Could you check a few things on this model? Use its own coordinates, in mm. A direction names the side the tool comes from. Coordinates: 2 decimals unless noted, no trailing zeros. Loops run counter-clockwise (first coordinate to the right, second up) from the corner with the lowest first, then second, coordinate; pieces in that order, holes last. Notation, with made-up numbers: (58.25, 33.25) -> (113.25, 33.25) arc R25 ccw to (113.25, 62.25) -> close; hole circle Ø9 at (79.25, -19.5). An arc over 180 degrees is marked (long way). One line per question, with ' | ' between items.
```python
from build123d import *

# Parameters (mm, degrees)
F0_W     = 32
F0_H     = 16
F1_DEPTH = 10
F2_R     = 2.5
F3_DEPTH = 2
F4_T     = -2
F5_R     = 3.75
F5_R_2   = 3.25
F6_DEPTH = 8
F8_DEPTH = 6.5


with BuildPart() as f1:
    # F0 (on Top) → F1 (new body)
    with BuildSketch(Plane.XY):
        Rectangle(F0_W, F0_H)
    extrude(amount=F1_DEPTH)

    # F2 (on face) → F3 (join)
    with BuildSketch(Plane.XY.offset(10)):
        with Locations((-11.5, 4)):
            Circle(F2_R)
        with Locations((-3.5, 4)):
            Circle(F2_R)
        with Locations((12.5, 4)):
            Circle(F2_R)
        with Locations((12.5, -4)):
            Circle(F2_R)
        with Locations((4.5, -4)):
            Circle(F2_R)
        with Locations((-3.5, -4)):
            Circle(F2_R)
        with Locations((-11.5, -4)):
            Circle(F2_R)
        with Locations((4.5, 4)):
            Circle(F2_R)
    extrude(amount=F3_DEPTH)

    # F4
    f4_openings = [f1.faces().sort_by_distance(p)[0] for p in [
        (0, 0, 0),
    ]]
    offset(amount=F4_T, openings=f4_openings, kind=Kind.INTERSECTION)

    # F5 (on face) → F6 (join, through all)
    with BuildSketch(Plane(origin=(0, 0, 8), x_dir=(1, 0, 0), z_dir=(0, 0, -1))):
        with Locations((-7.5, 0)):
            Circle(F5_R)
        with Locations((-7.5, 0)):
            Circle(F5_R_2, mode=Mode.SUBTRACT)
        with Locations((0.7, 0)):
            Circle(F5_R)
        with Locations((0.7, 0)):
            Circle(F5_R_2, mode=Mode.SUBTRACT)
        with Locations((8.9, 0)):
            Circle(F5_R)
        with Locations((8.9, 0)):
            Circle(F5_R_2, mode=Mode.SUBTRACT)
    extrude(amount=F6_DEPTH)

    # F7 (on face) → F8 (join)
    with BuildSketch(Plane(origin=(0, 0, 8), x_dir=(1, 0, 0), z_dir=(0, 0, -1))):
        with BuildLine():
            ThreePointArc((-1.3, 3.1721443851), (0.7, 3.75), (2.7, 3.1721443851))
            Line((2.7, 3.1721443851), (2.7, 6))
            Line((2.7, 6), (-1.3, 6))
            Line((-1.3, 6), (-1.3, 3.1721443851))
        make_face()
        with BuildLine():
            Line((2.7, -6), (2.7, -3.1721443851))
            ThreePointArc((2.7, -3.1721443851), (0.7, -3.75), (-1.3, -3.1721443851))
            Line((-1.3, -3.1721443851), (-1.3, -6))
            Line((-1.3, -6), (2.7, -6))
        make_face()
    extrude(amount=F8_DEPTH)


solid = f1.part
```
Q1. For faces 1 (the face through (-14, 4, 11)), 2 (the face through (-4, -4, 12)), 3 (the face through (-3.5, -4, 10)), which set-ups out of +Z, -Z, +X, -X, +Y, -Y let a thin tool reach every point of the face, with its end or its side?
Values follow:
face 1: +Z | face 2: +Z, +X, -X, +Y, -Y | face 3: -Z
Q2. We'd pull the mould along X, two halves only. Please class faces 4 (the face through (-2.064, -2.534, 4.056)), 5 (the face through (0, 7, 0)): released by +X, released by -X, zero draft, split by the parting line, or undercut.
Values follow:
face 4: undercut | face 5: zero draft
Q3. For pin 1 (3 mm diameter, centred on x = 1, y = -4.5, fed in from -Z); pin 2 (1.1 mm diameter, centred on x = 12.5, y = -4, fed in from -Z); pin 3 (0.5 mm diameter, centred on x = 4.5, y = 4, fed in from -Z), each with a flat end and sliding along its axis, tell me the tip position at first contact or that it passes through.
Values follow:
pin 1: stops at z = 0 | pin 2: stops at z = 8 | pin 3: stops at z = 10
Q4. Imagine slicing it at B-B on z = 10.5. Write out the boundary of the cut face in (x, y), plus the area to 3 significant figures.
Values follow:
outline: circle Ø5 at (-11.5, -4); circle Ø5 at (-11.5, 4); circle Ø5 at (-3.5, -4); circle Ø5 at (-3.5, 4); circle Ø5 at (4.5, -4); circle Ø5 at (4.5, 4); circle Ø5 at (12.5, -4); circle Ø5 at (12.5, 4) | area: 157 mm2
Q5. Please list where these lines run through material, in increasing order: L1, parallel to Y at x = 8.9, z = 2.5; L2, parallel to Y at x = 12.5, z = 9.05; L3, parallel to X at y = 4, z = 9.15. Write a range as [from, to].
Values follow:
L1: y = [-8, -6], [-3.75, -3.25], [3.25, 3.75], [6, 8] | L2: y = [-8, -4.5], [-3.5, 3.5], [4.5, 8] | L3: x = [-16, -12], [-11, -4], [-3, 4], [5, 12], [13, 16]
Q6. Imagine slicing it at A-A on z = 3.25. Write out the boundary of the cut face in (x, y).
Values follow:
outline: (-16, -8) -> (16, -8) -> (16, 8) -> (-16, 8) -> close; circle Ø7.5 at (-7.5, 0); circle Ø7.5 at (8.9, 0); hole (-14, -6) -> (-1.3, -6) -> (-1.3, -3.17) arc R3.75 cw to (-1.3, 3.17) -> (-1.3, 6) -> (-14, 6) -> close; hole circle Ø6.5 at (-7.5, 0); hole circle Ø6.5 at (0.7, 0); hole (2.7, -6) -> (14, -6) -> (14, 6) -> (2.7, 6) -> (2.7, 3.17) arc R3.75 cw to (2.7, -3.17) -> close; hole circle Ø6.5 at (8.9, 0)
Q7. Imagine slicing it at D-D on x = 0.7. Write out the boundary of the cut face in (y, z).
Values follow:
outline: (-8, 0) -> (-6, 0) -> (-6, 1.5) -> (-3.75, 1.5) -> (-3.75, 0) -> (-3.25, 0) -> (-3.25, 8) -> (3.25, 8) -> (3.25, 0) -> (3.75, 0) -> (3.75, 1.5) -> (6, 1.5) -> (6, 0) -> (8, 0) -> (8, 10) -> (-8, 10) -> close
